```python
from build123d import *

# Parameters (mm, degrees)
SKETCH_2_R          = 1.5
EXTRUDE_1_DEPTH     = 8
CUT_EXTRUDE_1_DEPTH = 2
CHAMFER_1_SIZE      = 0.2
FILLET_1_R          = 0.2


with BuildPart() as part:
    # 草图1 → 旋转1 (revolve)
    with BuildSketch(Plane.XY):
        Polygon((0, 0), (0, -2), (1.5, -2), (3, 0), align=None)
    revolve(axis=Axis((0, 0, 0), (0, -1, 0)))

    # 草图2 → 凸台-拉伸1 (add)
    with BuildSketch(Plane.XZ.offset(2)):
        Circle(SKETCH_2_R)
    extrude(amount=EXTRUDE_1_DEPTH)

    # 草图3 → 切除-拉伸1 (cut)
    with BuildSketch(Plane(origin=(0, 0, 0), x_dir=(1, 0, 0), z_dir=(0, 1, 0))):
        Polygon((-1.327905619, 0), (-0.66395281, -1.15), (0.66395281, -1.15), (1.327905619, 0), (0.66395281, 1.15), (-0.66395281, 1.15), align=None)
    extrude(amount=-CUT_EXTRUDE_1_DEPTH, mode=Mode.SUBTRACT)

    # 倒角1
    chamfer_1_edges = [part.edges().sort_by_distance(p)[0] for p in [
        (-1.5, -10, 0),
    ]]
    chamfer(chamfer_1_edges, length=CHAMFER_1_SIZE)

    # 圆角1
    fillet_1_edges = [part.edges().sort_by_distance(p)[0] for p in [
        (-3, 0, 0),
    ]]
    fillet(fillet_1_edges, radius=FILLET_1_R)


solid = part.part
```
Build history of the part. All positions in model axes, mm. A direction names the side the tool comes from. Give positions to 0.01 mm unless a question says otherwise; leave off trailing zeros. Loops run counter-clockwise (first coordinate to the right, second up) from the corner with the lowest first, then second, coordinate; pieces in that order, holes last.
Item 1: Flat gauge pins, fed straight in: pin 1 (1.5 mm diameter, centred on x = 0, y = -1, fed in from -Z); pin 2 (2 mm diameter, centred on x = -2, y = -2.5, fed in from +Z); pin 3 (1 mm diameter, centred on y = -3, z = 1, fed in from -X). Where does each tip first touch, or does it go through?
Answers follow:
pin 1: stops at z = -2.79
pin 2: stops at z = 1.12
pin 3: stops at x = -1.41
Item 2: Drill centre lines: line 1 (Y direction, x = 1.9, z = 0.7); line 2 (Y direction, x = 0.25, z = 0.65); line 3 (Z direction, x = 1.15, y = -0.25). Where is each one in solid material? Low to high.
Answers follow:
line 1: y = -1.3 to 0
line 2: y = -10 to -2
line 3: z = -2.55 to -0.31, 0.31 to 2.55
Item 3: Slice it at A-A, the plane x = 0. List the corners of the cut face in (y, z), and give its area (3 significant figures).
Answers follow:
outline: (-10, -1.3) - (-9.8, -1.5) - (-2, -1.5) - (-0.32, -2.76) arc R0.2 ccw to (0, -2.6) - (0, -1.15) - (-2, -1.15) - (-2, 1.15) - (0, 1.15) - (0, 2.6) arc R0.2 ccw to (-0.32, 2.76) - (-2, 1.5) - (-9.8, 1.5) - (-10, 1.3) - close
area: 28.3 mm2
Item 4: Pull direction X, two halves, no side cores. Call faces 3 (the face through (1, -0.99, -0.57)), 4 (the face through (-1.5, -5.85, 0.07)), 5 (the face through (1, 0, -1)), 6 (the face through (-1, -0.99, 0.57)): released by +X, released by -X, zero draft, split by the parting line, or undercut.
Answers follow:
face 3: undercut
face 4: split by the parting line
face 5: zero draft
face 6: undercut
Item 5: Which spindle directions (+Z, -Z, +X, -X, +Y, -Y) get a long thin tool onto all of the face, cutting with end or side? Do faces 1 (the face through (-0.991, -0.986, -0.583)), 2 (the face through (0, -10, 0)). Say none if no direction does.
Answers follow:
face 1: +Y
face 2: +Z, -Z, +X, -X, -Y
Item 6: Slice it at C-C, the plane y = -3.5. List the corners of the cut face in (x, z).
Answers follow:
outline: circle Ø3 at (0, 0)
